Source: CAD feature listing. Evaluate the final solid. Frame: model axes, mm. Coordinates: 2 decimals unless noted, no trailing zeros. Order: outer loops, then holes, each group sorted by start corner. A loop starts at its lowest first (then second) coordinate and runs counter-clockwise, first axis right, second up. Notation, with made-up numbers: (50, 73) - (76, 73) arc R13 cw to (76, 93) - close; hole circle Ø10 at (33, 30). An arc over 180 degrees is marked (long way). One line per question, with ' | ' between items.
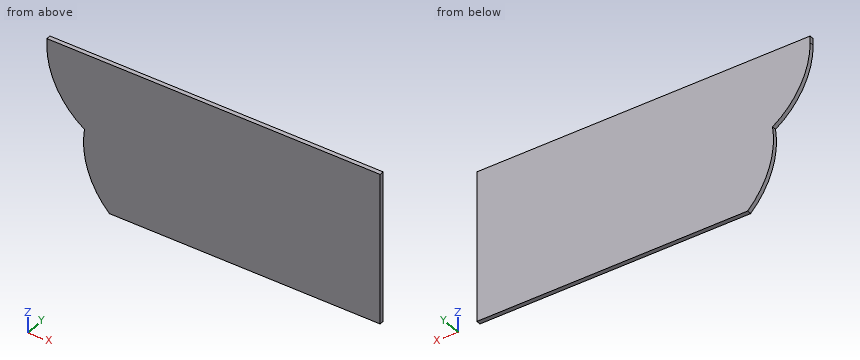
from build123d import *

# Parameters (mm, degrees)
F1_DEPTH = 15.875


with BuildPart() as f1:
    # F0 (on Front) → F1 (new body)
    with BuildSketch(Plane.XZ):
        with BuildLine():
            Line((1150.660626, -55.057509), (-68.539374, -55.057509))
            Line((-68.539374, -55.057509), (-68.539374, -80.457509))
            ThreePointArc((-68.539374, -80.457509), (-31.956463, -226.092789), (69.10691, -337.151958))
            ThreePointArc((69.10691, -337.151958), (81.782103, -486.286712), (160.060626, -613.857509))
            Line((160.060626, -613.857509), (1150.660626, -613.857509))
            Line((1150.660626, -613.857509), (1150.660626, -55.057509))
        make_face()
    extrude(amount=F1_DEPTH)


solid = f1.part
(1) Cut plane B-B (x = 104). Return the cut outline in (y, z) (1 decimal).
Taken from the geometry:
outline: (-15.9, -538.2) - (0, -538.2) - (0, -55.1) - (-15.9, -55.1) - close
(2) Cut plane C-C (z = -446). Return the cut outline in (x, y) (3 decimals), and give its area (3 significant figures).
Taken from the geometry:
outline: (71.35, -15.875) - (1150.661, -15.875) - (1150.661, 0) - (71.35, 0) - close | area: 17,100 mm²
(3) Cut plane A-A (y = -7.5). Return the cut outline in (x, z).
Taken from the geometry:
outline: (-68.54, -80.46) arc R308.18 ccw to (69.11, -337.15) arc R324.4 ccw to (160.06, -613.86) - (1150.66, -613.86) - (1150.66, -55.06) - (-68.54, -55.06) - close
(4) Material intervals for L1, parallel to X at y = -2.75, z = -88; L2, parallel to X at y = -12.25, z = -391; L3, parallel to Z at x = 28, y = -0.75, sorted ascending. Write a range as from..to.
Taken from the geometry:
L1: x = -68.45..1150.66 | L2: x = 65.62..1150.66 | L3: z = -304.47..-55.06
(5) Pin query (flat end, axial travel): P1, Ø4, axis at y = -9, z = -213, coming from the -X side; P2, Ø4, axis at y = -6, z = -120.5, coming from the -X side. Return the tip coordinate at first contact, or that it passes through.
Taken from the geometry:
P1: stops at x = -39.52 | P2: stops at x = -66.18
